Verification items for this drawing (mm, ordinates from the low corner). Coordinates: 2 decimals unless noted, no trailing zeros. Write each loop counter-clockwise with the first axis right and the second up, starting at its lowest first coordinate (ties: lowest second). Pieces come first, ordered by that corner, then holes. Notation, with made-up numbers: (48.5, 4) -> (80.5, 4) arc R17 ccw to (80.5, 12) -> close; hole circle Ø2 at (68, 52). An arc over 180 degrees is marked (long way). One line per question, with ' | ' between items.
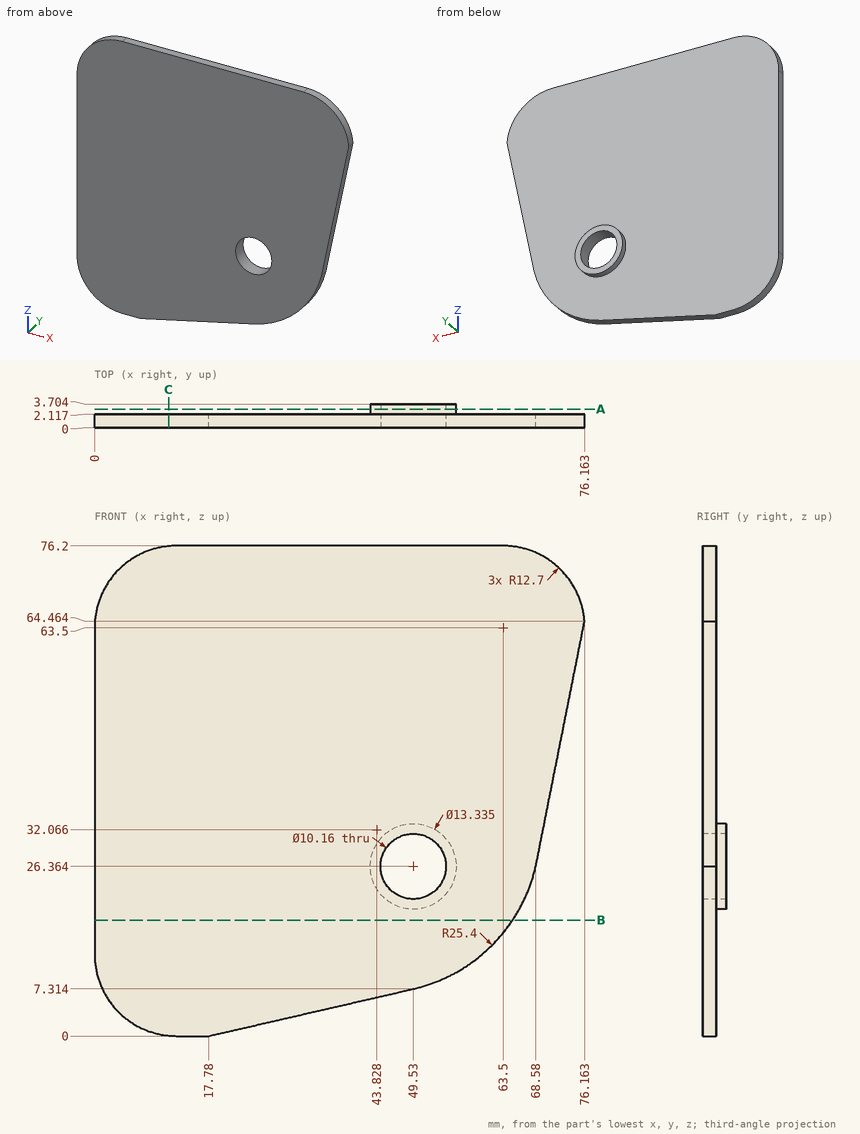
(1) Cross-section at B-B (z = 18). Record the cut outline in (x, y).
Answers below:
outline: (0, 0) -> (64.98, 0) -> (64.98, 2.12) -> (0, 2.12) -> close
(2) Material ranges on line 1 (Z direction, x = 49.53, y = 1); line 2 (Y direction, x = 52.5, z = 19); line 3 (Z direction, x = 49.53, y = 2.6), recorded low to high.
Answers below:
line 1: z = 7.31 to 21.28, 31.44 to 76.2 | line 2: y = 0 to 2.12 | line 3: z = 19.7 to 21.28, 31.44 to 33.03
(3) Cross-section at C-C (x = 11.5). Record the cut outline in (y, z), plus the area to 3 significant figures.
Answers below:
outline: (0, 0.06) -> (2.12, 0.06) -> (2.12, 76.14) -> (0, 76.14) -> close | area: 161 mm²
(4) Cross-section at A-A (y = 2.9). Record the cut outline in (x, z) (1 decimal).
Answers below:
outline: circle Ø13.3 at (49.5, 26.4); hole circle Ø10.2 at (49.5, 26.4)
(5) Depth check by flat-ended pin: P1, Ø4, axis at x = 59, z = 59, coming from the +Y side; P2, Ø1, axis at x = 26, y = 2.5, coming from the -Z side. Enter the tip coordinate at first touch or a pass-through.
Answers below:
P1: stops at y = 2.12 | P2: stops at z = 1.82
